Answer from the drawing. Dimensions are ordinates in mm from the lowest x, y and z of the part. A direction names the side the tool comes from. Coordinates: 2 decimals unless noted, no trailing zeros. Order: outer loops, then holes, each group sorted by start corner. A loop starts at its lowest first (then second) coordinate and runs counter-clockwise, first axis right, second up. Notation, with made-up numbers: M -32.75,-21.5 L 14.25,-21.5 A21 ccw 14.25,-13.5 Z; hole C 79,76.25 d9. An arc over 180 degrees is marked long. Write each question's results on one line, items separated by ' | '.
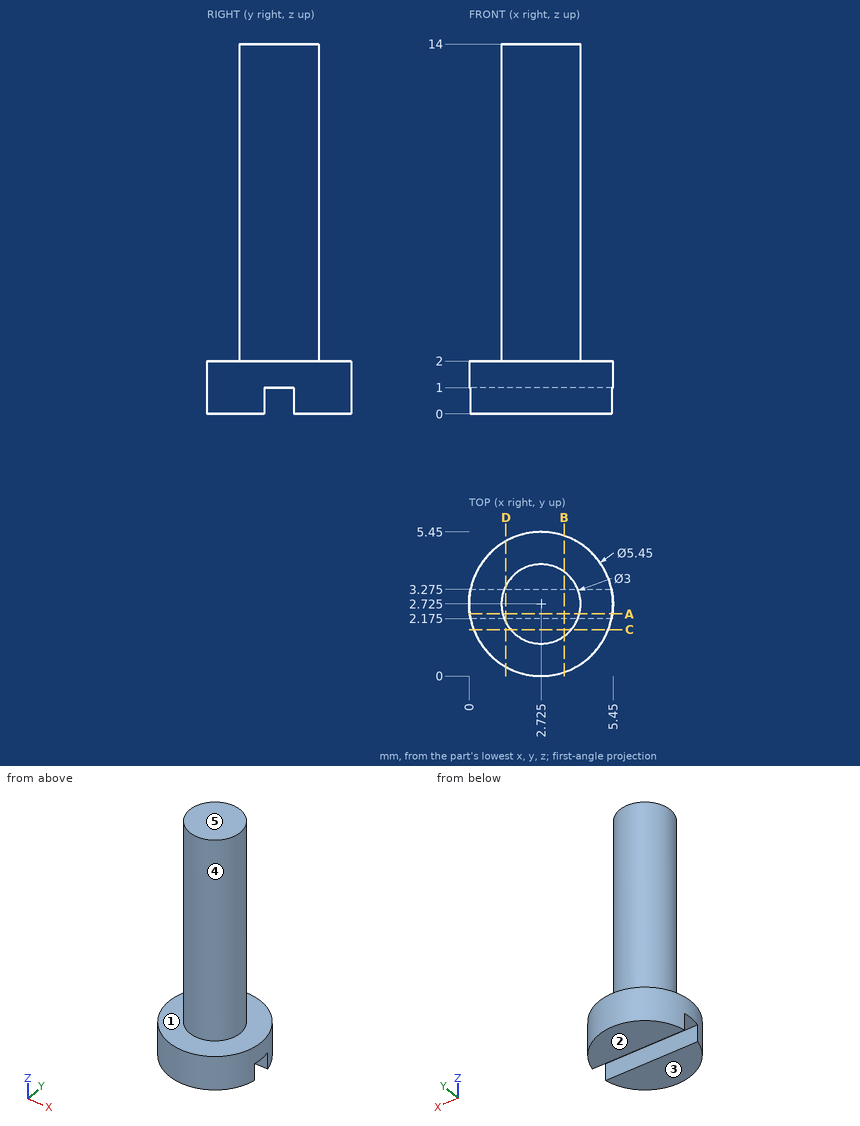
(1) For the marked faces 1 and 2, determine the directions among +Z, -Z, +X, -X, +Y, -Y from which every point of the face is accessible in a straight line to the end or side of a thin tool.
Conclusion:
face 1: +Z | face 2: -Z, +X, -X, +Y, -Y
(2) The part is cut by section A-A, the plane y = 2.35. Write down the section's boundary in (x, z), then the cut area to 3 significant figures.
Conclusion:
outline: M 0.03,1 L 5.42,1 L 5.42,2 L 4.18,2 L 4.18,14 L 1.27,14 L 1.27,2 L 0.03,2 Z | area: 40.3 mm²
(3) The part is cut by section D-D, the plane x = 1.4. Write down the section's boundary in (y, z) (3 decimals).
Conclusion:
outline: M 0.344,0 L 2.175,0 L 2.175,1 L 3.275,1 L 3.275,0 L 5.106,0 L 5.106,2 L 3.428,2 L 3.428,14 L 2.022,14 L 2.022,2 L 0.344,2 Z
(4) The mould has two halves that part along Z. Classify the marked faces 3, 4 and 5: pulls with the +Z half, pulls with the -Z half, needs draft (parallel to the pull), parting line crosses it, or undercut.
Conclusion:
face 3: pulls with the -Z half | face 4: needs draft | face 5: pulls with the +Z half
(5) The part is cut by section B-B, the plane x = 3.6. Write down the section's boundary in (y, z) (3 decimals), then the cut area to 3 significant figures.
Conclusion:
outline: M 0.144,0 L 2.175,0 L 2.175,1 L 3.275,1 L 3.275,0 L 5.306,0 L 5.306,2 L 3.943,2 L 3.943,14 L 1.507,14 L 1.507,2 L 0.144,2 Z | area: 38.5 mm²
(6) Straight lines are drawn through the part: line 1 (Z direction, x = 0.6, y = 4.2); line 2 (Z direction, x = 0.7, y = 2.4); line 3 (X direction, y = 1.7, z = 9). For each, find the intervals that lie inside material, in ascending order.
Conclusion:
line 1: 0 to 2 | line 2: 1 to 2 | line 3: 1.63 to 3.82
(7) The part is cut by section C-C, the plane y = 1.75. Write down the section's boundary in (x, z), then the cut area to 3 significant figures.
Conclusion:
outline: M 0.18,0 L 5.27,0 L 5.27,2 L 3.86,2 L 3.86,14 L 1.59,14 L 1.59,2 L 0.18,2 Z | area: 37.5 mm²
(8) Given pin 1 (0.5 mm diameter, centred on x = 4, z = 0.5, fed in from -Y); pin 2 (2 mm diameter, centred on x = 5, y = 1.5, fed in from +Z), each flat-ended and moving along its own axis, determine where each tip first touches the part or whether it passes through.
Conclusion:
pin 1: y = 0.2 | pin 2: z = 2
